Here's how the part is built. I have some questions about the finished solid (model axes, mm). A direction names the side the tool comes from. Round coordinates to 2 decimals unless told otherwise and drop trailing zeros. Loops run counter-clockwise (first coordinate to the right, second up) from the corner with the lowest first, then second, coordinate; pieces in that order, holes last. Notation, with made-up numbers: M -20.5,-21.5 L 14.5,-21.5 A37 cw 14.5,17.5 Z; hole C -28.5,18.5 d6. An arc over 180 degrees is marked long. One line per question, with ' | ' between items. Start each with the question number.
```python
from build123d import *

# Parameters (mm, degrees)
SKETCH_1_R          = 42.7
SKETCH_1_R_2        = 1.65
EXTRUDE_1_DEPTH     = 4
SKETCH_2_R          = 1
CUT_EXTRUDE_1_DEPTH = 4


with BuildPart() as part:
    # 草图1 → 凸台-拉伸1 (new body)
    with BuildSketch(Plane.XY):
        with BuildLine():
            ThreePointArc((-57.90455435, 8.325418039), (-56.664135325, 3.740040393), (-52.478752132, 1.493510837))
            ThreePointArc((-52.478752132, 1.493510837), (-51.965625699, -7.471529009), (-49.932223308, -16.217986173))
            ThreePointArc((-49.932223308, -16.217986173), (-53.315148558, -19.552674205), (-53.213471728, -24.301778261))
            ThreePointArc((-53.213471728, -24.301778261), (-49.690922522, -27.488622249), (-44.95538855, -27.115734184))
            ThreePointArc((-44.95538855, -27.115734184), (-39.676852654, -34.380188532), (-33.237553958, -40.63883619))
            ThreePointArc((-33.237553958, -40.63883619), (-34.280583312, -45.27310175), (-31.627487821, -49.213331671))
            ThreePointArc((-31.627487821, -49.213331671), (-26.941192918, -49.989841552), (-23.159006743, -47.115925192))
            ThreePointArc((-23.159006743, -47.115925192), (-14.790959234, -50.373381115), (-5.990196072, -52.157142857))
            ThreePointArc((-5.990196072, -52.157142857), (-4.36217508, -56.619639374), (0, -58.5))
            ThreePointArc((0, -58.5), (4.36217508, -56.619639374), (5.990196072, -52.157142857))
            ThreePointArc((5.990196072, -52.157142857), (14.790959234, -50.373381115), (23.159006743, -47.115925192))
            ThreePointArc((23.159006743, -47.115925192), (26.941192918, -49.989841552), (31.627487821, -49.213331671))
            ThreePointArc((31.627487821, -49.213331671), (34.280583312, -45.27310175), (33.237553958, -40.63883619))
            ThreePointArc((33.237553958, -40.63883619), (39.676852654, -34.380188532), (44.95538855, -27.115734184))
            ThreePointArc((44.95538855, -27.115734184), (49.690922522, -27.488622249), (53.213471728, -24.301778261))
            ThreePointArc((53.213471728, -24.301778261), (53.315148558, -19.552674205), (49.932223308, -16.217986173))
            ThreePointArc((49.932223308, -16.217986173), (51.965625699, -7.471529009), (52.478752132, 1.493510837))
            ThreePointArc((52.478752132, 1.493510837), (56.664135325, 3.740040393), (57.90455435, 8.325418039))
            ThreePointArc((57.90455435, 8.325418039), (55.422530843, 12.375589248), (50.773764562, 13.351959864))
            ThreePointArc((50.773764562, 13.351959864), (47.755679756, 21.809288183), (43.34048271, 29.62857672))
            ThreePointArc((43.34048271, 29.62857672), (45.646885531, 33.781266636), (44.2113501, 38.309352936))
            ThreePointArc((44.2113501, 38.309352936), (39.933651182, 40.374690556), (35.494994318, 38.682752984))
            ThreePointArc((35.494994318, 38.682752984), (28.383642916, 44.165810474), (20.441916256, 48.35677884))
            ThreePointArc((20.441916256, 48.35677884), (20.137072107, 53.097179409), (16.481354575, 56.130338956))
            ThreePointArc((16.481354575, 56.130338956), (11.766119429, 55.555112887), (8.946814173, 51.732045351))
            ThreePointArc((8.946814173, 51.732045351), (0, 52.5), (-8.946814173, 51.732045351))
            ThreePointArc((-8.946814173, 51.732045351), (-11.766119429, 55.555112887), (-16.481354575, 56.130338956))
            ThreePointArc((-16.481354575, 56.130338956), (-20.137072107, 53.097179409), (-20.441916256, 48.35677884))
            ThreePointArc((-20.441916256, 48.35677884), (-28.383642916, 44.165810474), (-35.494994318, 38.682752984))
            ThreePointArc((-35.494994318, 38.682752984), (-39.933651182, 40.374690556), (-44.2113501, 38.309352936))
            ThreePointArc((-44.2113501, 38.309352936), (-45.646885531, 33.781266636), (-43.34048271, 29.62857672))
            ThreePointArc((-43.34048271, 29.62857672), (-47.755679756, 21.809288183), (-50.773764562, 13.351959864))
            ThreePointArc((-50.773764562, 13.351959864), (-55.422530843, 12.375589248), (-57.90455435, 8.325418039))
        make_face()
        Circle(SKETCH_1_R, mode=Mode.SUBTRACT)
        with Locations((-51.965625699, 7.471529009)):
            Circle(SKETCH_1_R_2, mode=Mode.SUBTRACT)
        with Locations((-39.676852654, 34.380188532)):
            Circle(SKETCH_1_R_2, mode=Mode.SUBTRACT)
        with Locations((-14.790959234, 50.373381115)):
            Circle(SKETCH_1_R_2, mode=Mode.SUBTRACT)
        with Locations((14.790959234, 50.373381115)):
            Circle(SKETCH_1_R_2, mode=Mode.SUBTRACT)
        with Locations((39.676852654, 34.380188532)):
            Circle(SKETCH_1_R_2, mode=Mode.SUBTRACT)
        with Locations((51.965625699, 7.471529009)):
            Circle(SKETCH_1_R_2, mode=Mode.SUBTRACT)
        with Locations((47.755679756, -21.809288183)):
            Circle(SKETCH_1_R_2, mode=Mode.SUBTRACT)
        with Locations((28.383642916, -44.165810474)):
            Circle(SKETCH_1_R_2, mode=Mode.SUBTRACT)
        with Locations((0, -52.5)):
            Circle(SKETCH_1_R_2, mode=Mode.SUBTRACT)
        with Locations((-28.383642916, -44.165810474)):
            Circle(SKETCH_1_R_2, mode=Mode.SUBTRACT)
        with Locations((-47.755679756, -21.809288183)):
            Circle(SKETCH_1_R_2, mode=Mode.SUBTRACT)
    extrude(amount=EXTRUDE_1_DEPTH)

    # 草图2 → 切除-拉伸1 (cut)
    with BuildSketch(Plane.XY.offset(4)):
        with Locations((0, -42.7)):
            Circle(SKETCH_2_R)
        with Locations((0, 42.7)):
            Circle(SKETCH_2_R)
    extrude(amount=-CUT_EXTRUDE_1_DEPTH, mode=Mode.SUBTRACT)


solid = part.part
```
1) Imagine slicing it at C-C (z = 3.3). State how many separate pieces and enclosed holes the cut face has, then the cut area to 3 significant figures.
2) For faces 4 (the face through (46.107, -21.737, 1.972)), 5 (the face through (-14.91, -50.34, 1.97)), which set-ups out of +Z, -Z, +X, -X, +Y, -Y let a thin tool reach every point of the face, with its end or its side?
3) Imagine slicing it at B-B (x = 19). Write out the boundary of the cut face in (y, z), then the cut area to 3 significant figures.
4) Imagine slicing it at A-A (y = 0). Write out the boundary of the cut face in (x, z), then the cut area to 3 significant figures.
5) Please list where these lines run through material, in increasing order: L1, parallel to X at y = 35.5, z = 3.65; L2, parallel to Y at x = -27.5, z = 3.1; L3, parallel to Y at x = 46.5, z = 2.1. Write a range as from..to.
6) I'm going to push flat-ended pins straight in: pin 1 Ø5.5 at (x, y) = (39.68, 34.38) entering from -Z; pin 2 Ø1.5 at (x, z) = (-15.5, 2.5) entering from -Y; pin 3 Ø2 at (x, z) = (34.5, 2.5) entering from +Y. Where does each tip first touch, or does it pass through?
7) We'd pull the mould along X, two halves only. Please class faces 1 (the face through (51.948, -7.596, 1.972)), 2 (the face through (25, -35, 0)), 3 (the face through (42.69, -0.92, 1.97)): pulls with the +X half, pulls with the -X half, needs draft (parallel to the pull), parting line crosses it, or undercut.
Results are:
1) separate pieces: 1 | enclosed holes: 12 | area: 3,470 mm²
2) face 4: +Z, -Z | face 5: +Z, -Z, -Y
3) outline: M -48.94,0 L -38.24,0 L -38.24,4 L -48.94,4 Z; M 38.24,0 L 54.65,0 L 54.65,4 L 38.24,4 Z | area: 108 mm²
4) outline: M -52.5,0 L -42.7,0 L -42.7,4 L -52.5,4 Z; M 42.7,0 L 52.5,0 L 52.5,4 L 42.7,4 Z | area: 78.4 mm²
5) L1: -45.57..-40.89, -38.47..-23.73, 23.73..38.47, 40.89..45.57 | L2: -50.1..-45.56, -42.77..-32.67, 32.67..44.72 | L3: -27.68..-22.88, -20.74..24.37
6) pin 1: z = 0 | pin 2: y = -50.39 | pin 3: y = 40.42
7) face 1: pulls with the +X half | face 2: needs draft | face 3: undercut
